Answer from the drawing. Dimensions are ordinates in mm from the lowest x, y and z of the part. A direction names the side the tool comes from. Round coordinates to 2 decimals unless told otherwise and drop trailing zeros. Loops run counter-clockwise (first coordinate to the right, second up) from the corner with the lowest first, then second, coordinate; pieces in that order, holes last.
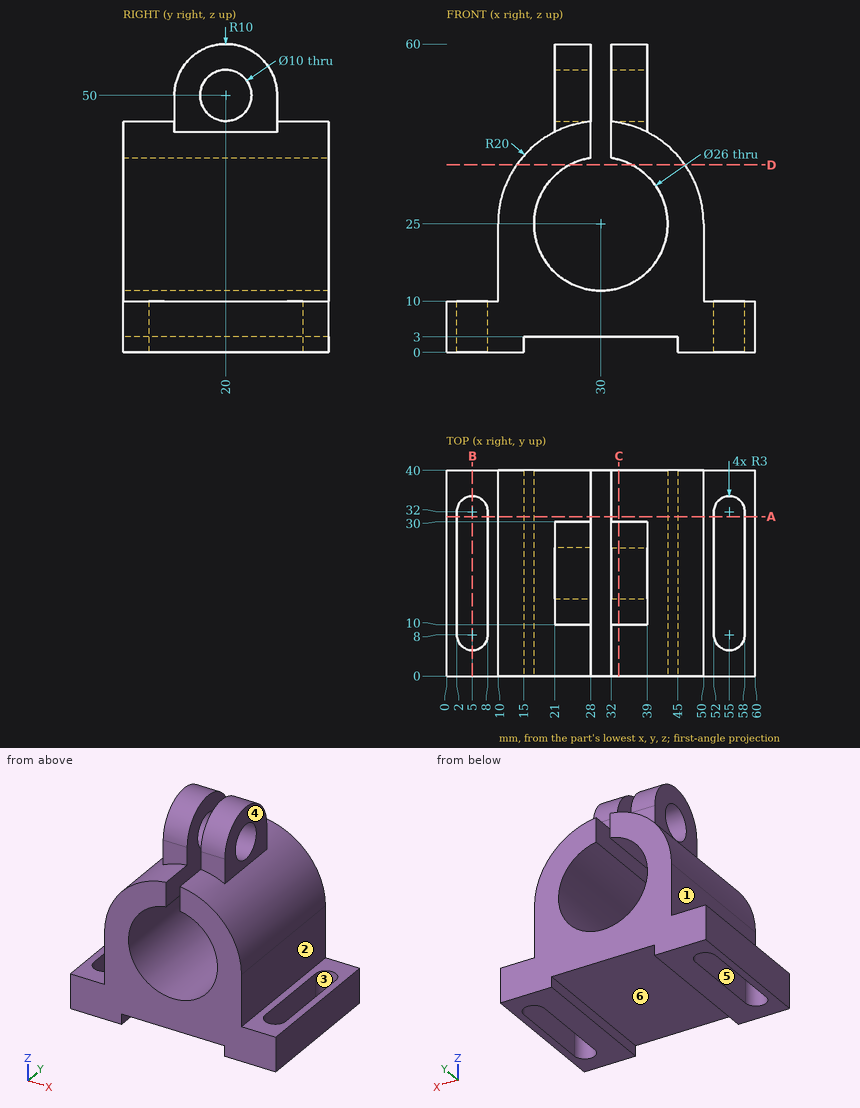
1. Which of the six approach directions +Z, -Z, +X, -X, +Y, -Y give full straight-line access (tool end or side, diameter ignored) to the marked faces 4, 5 and 6?
Answer key:
face 4: +Z, +X, +Y, -Y
face 5: +Z, -Z
face 6: -Z, +Y, -Y
2. Find section D-D (z = 36.5). Write down the section's boundary in (x, y).
Answer key:
outline: (13.64, 0) - (23.94, 0) - (23.94, 40) - (13.64, 40) - close; (36.06, 0) - (46.36, 0) - (46.36, 40) - (36.06, 40) - close
3. Consider probe 1 along X at (y, z) = (10, 25); probe 2 along Z at (x, y) = (23, 20); probe 3 along Z at (x, y) = (35.5, 20). Determine where each line is inside the solid, lowest interval first.
Answer key:
probe 1: x = 10 to 17, 43 to 50
probe 2: z = 3 to 14.05, 35.95 to 45, 55 to 60
probe 3: z = 3 to 13.22, 36.78 to 45, 55 to 60
4. Find section B-B (x = 5). Write down the section's boundary in (y, z).
Answer key:
outline: (0, 0) - (5, 0) - (5, 10) - (0, 10) - close; (35, 0) - (40, 0) - (40, 10) - (35, 10) - close
5. Find section C-C (x = 33.5). Write down the section's boundary in (y, z).
Answer key:
outline: (0, 3) - (40, 3) - (40, 12.48) - (0, 12.48) - close; (0, 37.52) - (40, 37.52) - (40, 44.69) - (30, 44.69) - (30, 50) arc R10 ccw to (10, 50) - (10, 44.69) - (0, 44.69) - close; hole circle Ø10 at (20, 50)
6. Find section A-A (y = 31). Write down the section's boundary in (x, z).
Answer key:
outline: (0, 0) - (2, 0) - (2, 10) - (0, 10) - close; (8, 0) - (15, 0) - (15, 3) - (45, 3) - (45, 0) - (52, 0) - (52, 10) - (50, 10) - (50, 25) arc R20 ccw to (32, 44.9) - (32, 37.85) arc R13 cw (long way) to (28, 37.85) - (28, 44.9) arc R20 ccw to (10, 25) - (10, 10) - (8, 10) - close; (58, 0) - (60, 0) - (60, 10) - (58, 10) - close
7. Given pin 1 (11 mm diameter, centred on x = 6, y = 12.5, fed in from +Z); pin 2 (7.5 mm diameter, centred on y = 16.5, z = 14.5, fed in from +X); pin 3 (11 mm diameter, centred on y = 15, z = 5, fed in from -X); pin 4 (4.5 mm diameter, centred on y = 24, z = 21, fed in from -X), each flat-ended and moving along its own axis, determine where each tip first touches the part or whether it passes through.
Answer key:
pin 1: stops at z = 32.6
pin 2: stops at x = 50
pin 3: stops at x = 0
pin 4: stops at x = 10
8. Determine the mould class of the marked faces 1, 2 and 3 for opening direction X: +X half, -X half, draft (parallel to the pull), parting line (faces both ways), or undercut.
Answer key:
face 1: -X half
face 2: +X half
face 3: undercut
